Geometry: final body of the model. Coordinates: model frame, mm. Face numbers are marked on the shaded views. A direction names the side the tool comes from. Coordinates: 2 decimals unless noted, no trailing zeros. Write each loop counter-clockwise with the first axis right and the second up, starting at its lowest first coordinate (ties: lowest second). Pieces come first, ordered by that corner, then holes. Notation, with made-up numbers: (11, 73) - (62, 73) arc R25 cw to (62, 108) - close; hole circle Ø6 at (34, 0). An arc over 180 degrees is marked (long way). Answer as a JSON object with one key per item and string values. Group by question number.
Item 1: Section A-A on y = -4. Return loops of the section in (x, z), and give its area (3 significant figures).
Item 2: First-contact query: pin 1 Ø3 at (y, z) = (2, 17.5) entering from -X; pin 2 Ø1.5 at (x, y) = (23, 0.5) entering from -Z; pin 3 Ø6 at (x, y) = (29, 2.5) entering from +Z (3 decimals). Flat tips, straight axial feed; report the tip coordinate or a pass-through.
Item 3: Set-up query: the marked faces 1, 2 and 3. Return all of +Z, -Z, +X, -X, +Y, -Y with unobstructed straight access to the full face (end or side cutting, diameter ignored); none if empty.
Item 4: Line query: line 1 along Z through (x, y) = (27.5, 2.5); line 2 along X through (y, z) = (2.75, -11); line 3 along Z through (x, y) = (-1, -3.5). Output: solid intervals per line, ascending. Write a range as from..to.
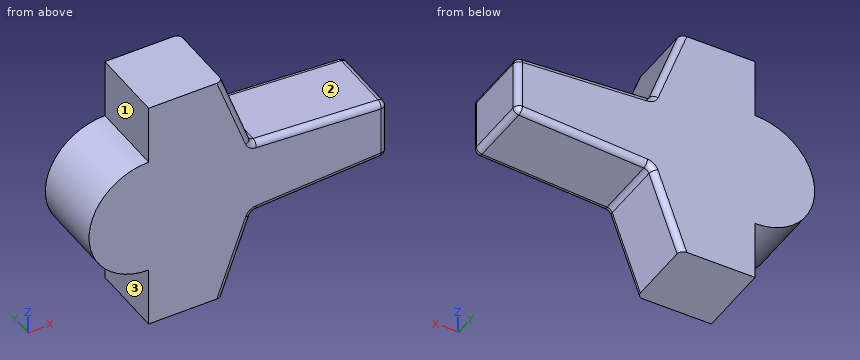
```python
from build123d import *

# Parameters (mm, degrees)
SKETCH1_R           = 10
BOSS_EXTRUDE1_DEPTH = 6.25
BOSS_EXTRUDE2_DEPTH = 6.25
BOSS_EXTRUDE5_DEPTH = 12.5
FILLET2_R           = 1
FILLET3_R           = 1


with BuildPart() as part:
    # Sketch1 → Boss-Extrude1 (new, symmetric)
    with BuildSketch(Plane(origin=(0, 0, 0), x_dir=(-1, 0, 0), z_dir=(0, 1, 0))):
        with Locations(Location((0, 0, 0), (0, 0, 90))):
            Circle(SKETCH1_R)
    extrude(amount=BOSS_EXTRUDE1_DEPTH, both=True)

    # Sketch2 → Boss-Extrude2 (add, symmetric)
    with BuildSketch(Plane(origin=(0, 0, 0), x_dir=(-1, 0, 0), z_dir=(0, 1, 0))):
        Polygon((0, 0), (0, 7.5), (-40, 5), (-40, -5), (0, -7.5), align=None)
    extrude(amount=BOSS_EXTRUDE2_DEPTH, both=True)

    # Sketch4 → Boss-Extrude5 (add, through all)
    with BuildSketch(Plane(origin=(0, 6.25, 0), x_dir=(1, 0, 0), z_dir=(0, 1, 0))):
        Polygon((19.779404685, 0), (12.5, -20), (0, -20), (0, 20), (12.5, 20), align=None)
    extrude(amount=-BOSS_EXTRUDE5_DEPTH)

    # Fillet2
    fillet2_edges = [part.edges().sort_by_distance(p)[0] for p in [
        (40, 0, -5),
        (40, 0, 5),
        (17.446503424, 0, -6.409593536),
        (17.446503424, 0, 6.409593536),
    ]]
    fillet(fillet2_edges, radius=FILLET2_R)

    # Fillet3
    fillet3_edges = [part.edges().sort_by_distance(p)[0] for p in [
        (14.86129541, -6.25, 13.512394182),
        (14.86129541, 6.25, 13.512394182),
        (28.58114172, 6.25, 5.713678643),
        (28.58114172, -6.25, 5.713678643),
        (28.58114172, -6.25, -5.713678643),
        (28.58114172, 6.25, -5.713678643),
        (14.86129541, -6.25, -13.512394182),
        (14.86129541, 6.25, -13.512394182),
        (40, -6.25, 0),
        (39.728827238, -6.25, 4.745246418),
        (39.728827238, -6.25, -4.745246418),
        (40, 6.25, 0),
        (39.728827238, 6.25, 4.745246418),
        (39.728827238, 6.25, -4.745246418),
        (17.563425222, -6.25, 6.565953441),
        (17.563425222, 6.25, 6.565953441),
        (17.563425222, 6.25, -6.565953441),
        (17.563425222, -6.25, -6.565953441),
    ]]
    fillet(fillet3_edges, radius=FILLET3_R)


solid = part.part
```
Checks:
{
 "1": {"outline": "(0, -20) - (12.5, -20) - (17.22, -7.02) arc R1 cw to (18.1, -6.37) - (39.06, -5.06) arc R1 ccw to (40, -4.06) - (40, 4.06) arc R1 ccw to (39.06, 5.06) - (18.1, 6.37) arc R1 cw to (17.22, 7.02) - (12.5, 20) - (0, 20) - (0, 10) arc R10 ccw to (0, -10) - close", "area": "1,040 mm^2"},
 "2": {"pin 1": "x = 0", "pin 2": "z = -6.11", "pin 3": "z = 5.875"},
 "3": {"face 1": "+Z, -X, +Y, -Y", "face 2": "+Z, +X, +Y, -Y", "face 3": "-Z, -X, +Y, -Y"},
 "4": {"line 1": "-5.78..5.78", "line 2": "0..15.78", "line 3": "-9.95..9.95"}
}
